```python
from build123d import *

# Parameters (mm, degrees)
F0_W     = 15.875
F0_H     = 15.875
F1_DEPTH = 38.1
F2_W     = 14.2875
F2_H     = 14.2875
F3_DEPTH = 76.2
F4_R     = 1.7859375
F5_DEPTH = 1.5875
F6_R     = 1.7859375
F7_DEPTH = 1.5875


with BuildPart() as f1:
    # F0 (on Top) → F1 (new body, symmetric)
    with BuildSketch(Plane.XY):
        Rectangle(F0_W, F0_H)
    extrude(amount=F1_DEPTH, both=True)

    # F2 (on face) → F3 (cut)
    with BuildSketch(Plane.XY.offset(38.1)):
        with Locations((-0.79375, 0.79375)):
            Rectangle(F2_W, F2_H)
    extrude(amount=-F3_DEPTH, mode=Mode.SUBTRACT)

    # F4 (on face) → F5 (cut, through all)
    with BuildSketch(Plane.XZ.offset(7.9375)):
        with Locations((0, -25.4)):
            Circle(F4_R)
        with Locations((0, 25.4)):
            Circle(F4_R)
    extrude(amount=-F5_DEPTH, mode=Mode.SUBTRACT)

    # F6 (on face) → F7 (cut, through all)
    with BuildSketch(Plane.YZ.offset(7.9375)):
        with Locations((0, -19.05)):
            Circle(F6_R)
        with Locations((0, 19.05)):
            Circle(F6_R)
    extrude(amount=-F7_DEPTH, mode=Mode.SUBTRACT)


solid = f1.part
```
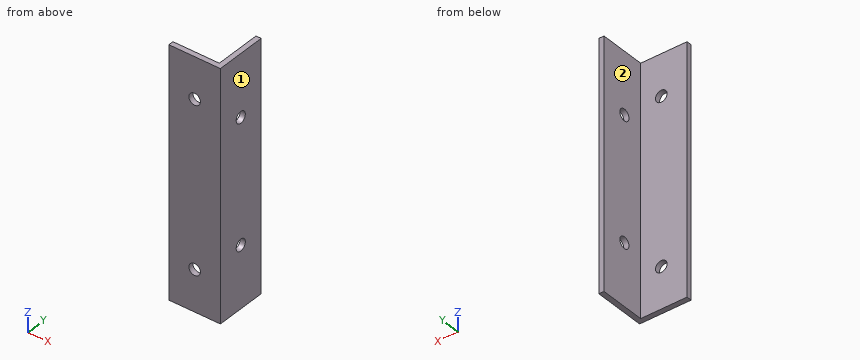
Can you work these out from the model? Positions are in its coordinate system, mm. Face numbers are marked on the shaded views. A direction names the side the tool comes from. Give positions to 0.01 mm unless a question says otherwise; leave off trailing zeros. Order: outer loops, then holes, each group sorted by start corner. A loop starts at its lowest first (then second) coordinate and runs counter-clockwise, first axis right, second up. Notation, with made-up numbers: (12, 38) - (32, 38) arc R30 ccw to (32, 72) - close; hole circle Ø11 at (-13.5, 86.25). An arc over 180 degrees is marked (long way). Use a Markdown table: item, result. Add a question column.
Q1. Please list where these lines run through material, in increasing order: line 1 along Z through (x, y) = (7.5, 0); line 2 along X through (y, z) = (0, -14.5); line 3 along Y through (x, z) = (-6.25, 27).
Q2. If we section it at C-C on y = 0.5: Write out the boundary of the cut face in (x, z), plus the area to 3 significant figures.
Q3. If we section it at A-A on x = 0: Write out the boundary of the cut face in (y, z), plus the area to 3 significant figures.
Q4. On a 3-axis mill with a long thin cutter (end or side, diameter ignored), from which of +Z, -Z, +X, -X, +Y, -Y can I reach the whole of each face in a straight line? I mean the marked faces 1 and 2. Say none if no direction works.
Q5. I'm going to push flat-ended pins straight in: pin 1 (4.5 mm diameter, centred on x = 0, z = 25.4, fed in from +Y); pin 2 (8 mm diameter, centred on y = 2, z = 10.5, fed in from -X); pin 3 (5 mm diameter, centred on x = 1, y = -5.5, fed in from -Z). Where does each tip first touch, or does it pass through?
Q6. If we section it at D-D on z = 31: Write out the boundary of the cut face in (x, y).
Q7. If we section it at B-B on z = -25.4: Write out the boundary of the cut face in (x, y), plus the area to 3 significant figures.
Answers follow:
| question | item | result |
|---|---|---|
| 1 | line 1 | z = -38.1 to -20.84, -17.26 to 17.26, 20.84 to 38.1 |
| 1 | line 2 | x = 6.35 to 7.94 |
| 1 | line 3 | y = -7.94 to -6.35 |
| 2 | outline | (6.35, -38.1) - (7.94, -38.1) - (7.94, -20.76) - (6.35, -20.76) - close; (6.35, -17.34) - (7.94, -17.34) - (7.94, 17.34) - (6.35, 17.34) - close; (6.35, 20.76) - (7.94, 20.76) - (7.94, 38.1) - (6.35, 38.1) - close |
| 2 | area | 110 mm^2 |
| 3 | outline | (-7.94, -38.1) - (-6.35, -38.1) - (-6.35, -27.19) - (-7.94, -27.19) - close; (-7.94, -23.61) - (-6.35, -23.61) - (-6.35, 23.61) - (-7.94, 23.61) - close; (-7.94, 27.19) - (-6.35, 27.19) - (-6.35, 38.1) - (-7.94, 38.1) - close |
| 3 | area | 110 mm^2 |
| 4 | face 1 | +Z, -Z, +X, +Y, -Y |
| 4 | face 2 | +Z, -Z, -X, +Y |
| 5 | pin 1 | stops at y = -6.35 |
| 5 | pin 2 | stops at x = 6.35 |
| 5 | pin 3 | stops at z = -38.1 |
| 6 | outline | (-7.94, -7.94) - (7.94, -7.94) - (7.94, 7.94) - (6.35, 7.94) - (6.35, -6.35) - (-7.94, -6.35) - close |
| 7 | outline | (-7.94, -7.94) - (-1.79, -7.94) - (-1.79, -6.35) - (-7.94, -6.35) - close; (1.79, -7.94) - (7.94, -7.94) - (7.94, 7.94) - (6.35, 7.94) - (6.35, -6.35) - (1.79, -6.35) - close |
| 7 | area | 42.2 mm^2 |
